Model file for the job. Use its own axes, mm. Face numbers are marked on the shaded views. A direction names the side the tool comes from. Round coordinates to 2 decimals unless told otherwise and drop trailing zeros. Order: outer loops, then holes, each group sorted by start corner. A loop starts at its lowest first (then second) coordinate and runs counter-clockwise, first axis right, second up. Notation, with made-up numbers: (88, 68) - (96, 68) arc R18 cw to (96, 89) - close; hole circle Ø4 at (-19.75, 60). An arc over 180 degrees is marked (long way). Write item = value, one per line.
```python
from build123d import *

# Parameters (mm, degrees)
F1_DEPTH = 24
F3_DEPTH = 24
F5_DEPTH = 24
F6_R     = 5


with BuildPart() as f1:
    # F0 (on Top) → F1 (new body, symmetric)
    with BuildSketch(Plane.XY):
        Polygon((572.287187, -24), (600, 24), (-600, 24), (-572.287187, -24), align=None)
    extrude(amount=F1_DEPTH, both=True)

    # F2 (on face) → F3 (cut)
    with BuildSketch(Plane.XY.offset(24)):
        Polygon((544.574374, 24), (516.861561, -24), (572.287187, -24), (600, 24), align=None)
    extrude(amount=-F3_DEPTH, mode=Mode.SUBTRACT)

    # F4 (on face) → F5 (cut)
    with BuildSketch(Plane(origin=(0, 0, -24), x_dir=(1, 0, 0), z_dir=(0, 0, -1))):
        Polygon((-544.574374, -24), (-516.861561, 24), (-572.287187, 24), (-600, -24), align=None)
    extrude(amount=-F5_DEPTH, mode=Mode.SUBTRACT)

    # F6
    f6_edges = [f1.edges().sort_by_distance(p)[0] for p in [
        (27.712813, 24, -24),
        (27.712813, -24, -24),
    ]]
    fillet(f6_edges, radius=F6_R)


solid = f1.part
```
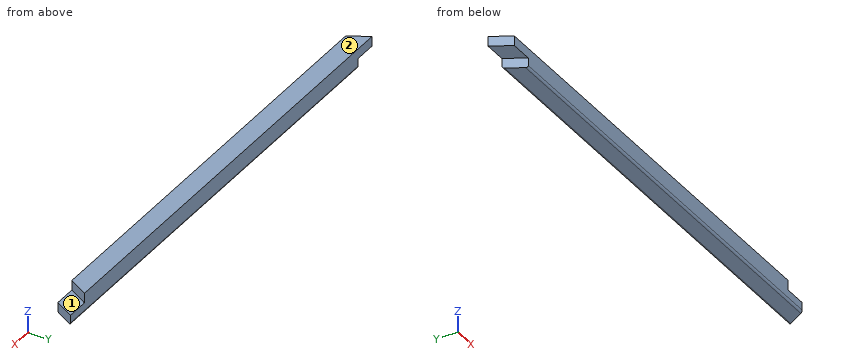
1) Cut at B-B (z = 9). Write the cut outline in (x, y).
Conclusion:
outline = (-600, 24) - (-572.29, -24) - (516.86, -24) - (544.57, 24) - close
2) Cut at A-A (y = -7). Write the cut outline in (x, z), and give its area (3 significant figures).
Conclusion:
outline = (-582.1, 0) - (-526.68, 0) - (-526.68, -24) - (582.1, -24) - (582.1, 0) - (526.68, 0) - (526.68, 24) - (-582.1, 24) - close
area = 53,200 mm^2
3) 3-axis set-ups, long thin cutter, end or side, ignore diameter. For the marked faces 1 and 2: which of +Z, -Z, +X, -X, +Y, -Y reach the whole face in a straight line?
Conclusion:
face_1 = +Z, +X, -Y
face_2 = +Z, +X, -X, +Y, -Y
4) Flat gauge pins, fed straight in: pin 1 Ø1 at (y, z) = (1.5, -1.5) entering from -X; pin 2 Ø3 at (y, z) = (-18.5, 3.5) entering from -X. Where does each tip first touch, or does it go through?
Conclusion:
pin_1 = -531.87
pin_2 = -576.33
5) Wall check: line 1 along Y through (x, z) = (507.5, -20.5); line 2 along X through (y, z) = (6.5, -4); line 3 along X through (y, z) = (-12.5, 10.5). Give the ranges that are in metal, low to high.
Conclusion:
line_1 = -23.77 to 23.77
line_2 = -534.47 to 589.9
line_3 = -578.93 to 523.5
